```python
from build123d import *

# Parameters (mm, degrees)
BOSS_EXTRU_1_DEPTH = 29
ESQUISSE2_W        = 18.5
ESQUISSE2_H        = 26
BOSS_EXTRU_2_DEPTH = 10
ESQUISSE3_W        = 18.5
ESQUISSE3_H        = 26
BOSS_EXTRU_3_DEPTH = 10
CONG_3_R           = 7
CONG_4_R           = 7
CONG_5_R           = 7
CONG_6_R           = 0.5
CONG_7_R           = 0.5
CONG_8_R           = 0.25


with BuildPart() as part:
    # Esquisse1 → Boss.-Extru.1 (new body)
    with BuildSketch(Plane.XY):
        Polygon((0, 0), (3, 0), (3, -23), (15.5, -23), (15.5, 0), (18.5, 0), (18.5, -26), (0, -26), align=None)
    extrude(amount=BOSS_EXTRU_1_DEPTH)

    # Esquisse2 → Boss.-Extru.2 (add)
    with BuildSketch(Plane(origin=(0, 0, 0), x_dir=(-1, 0, 0), z_dir=(0, 0, -1))):
        with Locations((-9.25, -13)):
            Rectangle(ESQUISSE2_W, ESQUISSE2_H)
    extrude(amount=BOSS_EXTRU_2_DEPTH)

    # Esquisse3 → Boss.-Extru.3 (add)
    with BuildSketch(Plane.XY.offset(29)):
        with Locations((9.25, -13)):
            Rectangle(ESQUISSE3_W, ESQUISSE3_H)
    extrude(amount=BOSS_EXTRU_3_DEPTH)

    # Congé3
    cong_3_edges = [part.edges().sort_by_distance(p)[0] for p in [
        (9.25, -26, 39),
    ]]
    fillet(cong_3_edges, radius=CONG_3_R)

    # Congé4
    cong_4_edges = [part.edges().sort_by_distance(p)[0] for p in [
        (18.5, -9.5, 39),
        (18.5, -26, 11),
        (18.5, -23.949747468, 36.949747468),
    ]]
    fillet(cong_4_edges, radius=CONG_4_R)

    # Congé5
    cong_5_edges = [part.edges().sort_by_distance(p)[0] for p in [
        (0, -9.5, 39),
        (0, -26, 11),
        (0, -23.949747468, 36.949747468),
    ]]
    fillet(cong_5_edges, radius=CONG_5_R)

    # Congé6
    cong_6_edges = [part.edges().sort_by_distance(p)[0] for p in [
        (18.5, -9.5, -10),
        (9.25, -26, -10),
        (16.449747468, -23.949747468, -10),
        (0, -9.5, -10),
        (2.050252532, -23.949747468, -10),
    ]]
    fillet(cong_6_edges, radius=CONG_6_R)

    # Congé7
    cong_7_edges = [part.edges().sort_by_distance(p)[0] for p in [
        (9.25, 0, 39),
        (18.5, 0, 11.25),
        (16.449747468, 0, 36.949747468),
        (0, 0, 11.25),
        (2.050252532, 0, 36.949747468),
        (9.25, 0, -10),
        (0.146446609, 0, -9.853553391),
        (18.353553391, 0, -9.853553391),
    ]]
    fillet(cong_7_edges, radius=CONG_7_R)

    # Congé8
    cong_8_edges = [part.edges().sort_by_distance(p)[0] for p in [
        (3, 0, 14.5),
        (3, -23, 14.5),
        (15.5, -23, 14.5),
        (15.5, 0, 14.5),
        (15.5, -11.5, 29),
        (9.25, -23, 29),
        (3, -11.5, 29),
        (9.25, 0, 0),
        (9.25, 0, 29),
        (9.25, -23, 0),
        (15.5, -11.5, 0),
    ]]
    fillet(cong_8_edges, radius=CONG_8_R)


solid = part.part
```
Input: part model. Units: mm. Frame: model coordinates. A direction names the side the tool comes from. Coordinates: 2 decimals unless noted, no trailing zeros. Loops run counter-clockwise (first coordinate to the right, second up) from the corner with the lowest first, then second, coordinate; pieces in that order, holes last. Notation, with made-up numbers: (49.25, 65) - (95.25, 65) arc R19 cw to (95.25, 102) - close; hole circle Ø9 at (26, 35). An arc over 180 degrees is marked (long way). Answer in a Markdown table with one row per item.
(1) Mould query, pull axis Z, two halves, no side actions, for faces 3 (the face through (9, -11, 29)), 4 (the face through (9.3, -24, 36.9)), 5 (the face through (9, -11, 0)), 6 (the face through (2.1, -24, 11.5)). Classes: pulls with the +Z half, pulls with the -Z half, needs draft (parallel to the pull), parting line crosses it, or undercut.
Model answer:
| item | result |
|---|---|
| face 3 | undercut |
| face 4 | pulls with the +Z half |
| face 5 | undercut |
| face 6 | needs draft |
(2) Cut plane B-B on z = 31. Output: boundary loops of the cut face in (x, y).
Model answer:
| item | result |
|---|---|
| outline | (0, -19) arc R7 ccw to (7, -26) - (11.5, -26) arc R7 ccw to (18.5, -19) - (18.5, -0.5) arc R0.5 ccw to (18, 0) - (0.5, 0) arc R0.5 ccw to (0, -0.5) - close |
(3) Cut plane D-D on z = 3. Output: boundary loops of the cut face in (x, y), plus the area to 3 significant figures.
Model answer:
| item | result |
|---|---|
| outline | (0, -19) arc R7 ccw to (7, -26) - (11.5, -26) arc R7 ccw to (18.5, -19) - (18.5, -0.5) arc R0.5 ccw to (18, 0) - (15.75, 0) arc R0.25 ccw to (15.5, -0.25) - (15.5, -22.75) arc R0.25 cw to (15.25, -23) - (3.25, -23) arc R0.25 cw to (3, -22.75) - (3, -0.25) arc R0.25 ccw to (2.75, 0) - (0.5, 0) arc R0.5 ccw to (0, -0.5) - close |
| area | 172 mm² |
(4) Cut plane C-C on x = 10.5. Output: boundary loops of the cut face in (y, z).
Model answer:
| item | result |
|---|---|
| outline | (-26, -9.5) arc R0.5 ccw to (-25.5, -10) - (-0.5, -10) arc R0.5 ccw to (0, -9.5) - (0, -0.25) arc R0.25 ccw to (-0.25, 0) - (-22.75, 0) arc R0.25 cw to (-23, 0.25) - (-23, 28.75) arc R0.25 cw to (-22.75, 29) - (-0.25, 29) arc R0.25 ccw to (0, 29.25) - (0, 38.5) arc R0.5 ccw to (-0.5, 39) - (-19, 39) arc R7 ccw to (-26, 32) - close |
(5) Cut plane A-A on y = -2.5. Output: boundary loops of the cut face in (x, z), plus the area to 3 significant figures.
Model answer:
| item | result |
|---|---|
| outline | (0, -9.5) arc R0.5 ccw to (0.5, -10) - (18, -10) arc R0.5 ccw to (18.5, -9.5) - (18.5, 32) arc R7 ccw to (11.5, 39) - (7, 39) arc R7 ccw to (0, 32) - close; hole (3, 0) - (15.25, 0) arc R0.25 ccw to (15.5, 0.25) - (15.5, 28.75) arc R0.25 ccw to (15.25, 29) - (3.25, 29) arc R0.25 ccw to (3, 28.75) - close |
| area | 523 mm² |
(6) Material intervals for L1, parallel to X at y = -17, z = 21.5; L2, parallel to Z at x = 9.5, y = -4.25; L3, parallel to Z at x = 5, y = -2.25, sorted ascending. Write a range as from..to.
Model answer:
| item | result |
|---|---|
| L1 | x = 0..3, 15.5..18.5 |
| L2 | z = -10..0, 29..39 |
| L3 | z = -10..0, 29..38.71 |
(7) Set-up query: faces 1 (the face through (9, -10, 39)), 2 (the face through (9, -23, 14)). Return all of +Z, -Z, +X, -X, +Y, -Y with unobstructed straight access to the full face (end or side cutting, diameter ignored); none if empty.
Model answer:
| item | result |
|---|---|
| face 1 | +Z, +X, -X, +Y, -Y |
| face 2 | +Y |
(8) Pin query (flat end, axial travel): P1, Ø6, axis at x = 12, z = 2, coming from the -Y side; P2, Ø6, axis at x = 16, z = 16.5, coming from the -Y side; P3, Ø1.5, axis at x = 5.5, y = -18, coming from the +Z side; P4, Ø3, axis at x = 2, z = 17, coming from the -Y side. Return the tip coordinate at first contact, or that it passes through.
Model answer:
| item | result |
|---|---|
| P1 | stops at y = -26 |
| P2 | stops at y = -25.84 |
| P3 | stops at z = 38.96 |
| P4 | stops at y = -25.06 |
